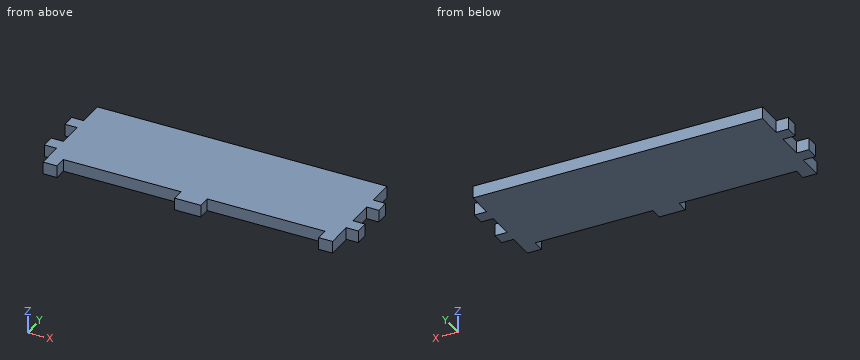
from build123d import *

# Parameters (mm, degrees)
BASE_SKETCH_W           = 304.8
BASE_SKETCH_H           = 89.79
BOSS_EXTRUDE1_DEPTH     = 11.81
JOINT_X_W               = 25.4
JOINT_X_H               = 11.81
BOSS_EXTRUDE2_DEPTH     = 11.81
JOINT_Y_W               = 11.81
JOINT_Y_H               = 25.4
CUT_EXTRUDE1_DEPTH      = 705.310070992
LPATTERN1_COUNT         = 3
LPATTERN1_PITCH         = 139.7
LPATTERN2_COUNT         = 3
LPATTERN2_PITCH         = 38.1
MIRROR1_COPY_1_SKETCH_W = 11.81
MIRROR1_COPY_1_SKETCH_H = 25.4
MIRROR1_COPY_1_DEPTH    = 705.310070992
MIRROR1_COPY_2_SKETCH_W = 11.81
MIRROR1_COPY_2_SKETCH_H = 25.4
MIRROR1_COPY_2_DEPTH    = 705.310070992


with BuildPart() as part:
    # Base_Sketch → Boss-Extrude1 (new body)
    with BuildSketch(Plane.XY):
        with Locations((-535.138681284, -95.622810132)):
            Rectangle(BASE_SKETCH_W, BASE_SKETCH_H)
    extrude(amount=BOSS_EXTRUDE1_DEPTH)

    # Joint_X → Boss-Extrude2 (add)
    with BuildSketch(Plane.XY.offset(11.81)):
        with Locations((-674.838681284, -146.422810132)):
            Rectangle(JOINT_X_W, JOINT_X_H)
    boss_extrude2 = extrude(amount=-BOSS_EXTRUDE2_DEPTH)

    # Joint_Y → Cut-Extrude1 (cut, through all)
    with BuildSketch(Plane.XY.offset(11.81)):
        with Locations((-681.633681284, -139.627810132)):
            Rectangle(JOINT_Y_W, JOINT_Y_H)
    cut_extrude1 = extrude(amount=-CUT_EXTRUDE1_DEPTH, mode=Mode.SUBTRACT)

    # LPattern1: Boss-Extrude2 ×3
    with Locations(*[(i * LPATTERN1_PITCH, 0, 0) for i in range(1, LPATTERN1_COUNT)]):
        add(boss_extrude2)

    # LPattern2: Cut-Extrude1 ×3
    with Locations(*[(0, i * LPATTERN2_PITCH, 0) for i in range(1, LPATTERN2_COUNT)]):
        add(cut_extrude1, mode=Mode.SUBTRACT)

    # Mirror1: Cut-Extrude1 across plane
    add(cut_extrude1.mirror(Plane.ZY.offset(535.138681284)), mode=Mode.SUBTRACT)

    # Mirror1 copy 1 sketch → Mirror1 copy 1 (cut, through all)
    with BuildSketch(Plane(origin=(-1070.277362567, 38.1, 11.81), x_dir=(-1, 0, 0), z_dir=(0, 0, 1))):
        with Locations((-681.633681284, 139.627810132)):
            Rectangle(MIRROR1_COPY_1_SKETCH_W, MIRROR1_COPY_1_SKETCH_H)
    extrude(amount=-MIRROR1_COPY_1_DEPTH, mode=Mode.SUBTRACT)

    # Mirror1 copy 2 sketch → Mirror1 copy 2 (cut, through all)
    with BuildSketch(Plane(origin=(-1070.277362567, 76.2, 11.81), x_dir=(-1, 0, 0), z_dir=(0, 0, 1))):
        with Locations((-681.633681284, 139.627810132)):
            Rectangle(MIRROR1_COPY_2_SKETCH_W, MIRROR1_COPY_2_SKETCH_H)
    extrude(amount=-MIRROR1_COPY_2_DEPTH, mode=Mode.SUBTRACT)


solid = part.part
CAD build for the part. Positions are in the model's coordinates, mm. Round coordinates to 2 decimals unless told otherwise and drop trailing zeros. Write each loop counter-clockwise with the first axis right and the second up, starting at its lowest first coordinate (ties: lowest second). Pieces come first, ordered by that corner, then holes. Notation, with made-up numbers: M 84.25,81.25 L 115.25,81.25 A28 cw 115.25,99.25 Z; hole C 65,-20 d6. An arc over 180 degrees is marked long. Put each result on its own line as item: value. Start each with the question number.
1) Saw through at C-C, the plane y = -95.5. Write the cut outline in (x, z), and give its area (3 significant figures).
2) Saw through at A-A, the plane z = 7.75. Write the cut outline in (x, y), and give its area (3 significant figures).
3) Pin check, flat tips, straight feed: pin 1 Ø8 at (x, y) = (-607, -90) entering from -Z; pin 2 Ø6 at (y, z) = (-103.5, 7.5) entering from -X; pin 3 Ø3.5 at (x, z) = (-684.5, 4) entering from +Y; pin 4 Ø6 at (x, z) = (-386, 7) entering from -Y. Stop position of each tip, or through.
4) Saw through at B-B, the plane x = -516. Write the cut outline in (y, z), and give its area (3 significant figures).
5) Drill centre lines: probe 1 along X at (y, z) = (-145, 7.25); probe 2 along Y at (x, z) = (-424, 9); probe 3 along X at (y, z) = (-98, 10.75). Where is each one in solid material? Low to high. Write a range as [from, to].
Resolved:
1. outline: M -675.73,0 L -394.55,0 L -394.55,11.81 L -675.73,11.81 Z
1. area: 3,320 mm²
2. outline: M -687.54,-126.93 L -675.73,-126.93 L -675.73,-152.33 L -662.14,-152.33 L -662.14,-140.52 L -547.84,-140.52 L -547.84,-152.33 L -522.44,-152.33 L -522.44,-140.52 L -408.14,-140.52 L -408.14,-152.33 L -394.55,-152.33 L -394.55,-126.93 L -382.74,-126.93 L -382.74,-114.23 L -394.55,-114.23 L -394.55,-88.83 L -382.74,-88.83 L -382.74,-76.13 L -394.55,-76.13 L -394.55,-50.73 L -675.73,-50.73 L -675.73,-76.13 L -687.54,-76.13 L -687.54,-88.83 L -675.73,-88.83 L -675.73,-114.23 L -687.54,-114.23 Z
2. area: 26,500 mm²
3. pin 1: z = 0
3. pin 2: x = -675.73
3. pin 3: y = -76.13
3. pin 4: y = -126.93
4. outline: M -140.52,0 L -50.73,0 L -50.73,11.81 L -140.52,11.81 Z
4. area: 1,060 mm²
5. probe 1: [-675.73, -662.14], [-547.84, -522.44], [-408.14, -394.55]
5. probe 2: [-140.52, -50.73]
5. probe 3: [-675.73, -394.55]
